from build123d import *

# Parameters (mm, degrees)
BOSS_EXTRUDE1_DEPTH = 30
SKETCH2_R           = 1.75
CUT_EXTRUDE2_DEPTH  = 42.231056256
CUT_EXTRUDE3_DEPTH  = 40.862263024
SKETCH5_W           = 33.611871568
SKETCH5_H           = 10
CUT_EXTRUDE4_DEPTH  = 42.231056256


with BuildPart() as part:
    # Sketch1 → Boss-Extrude1 (new body)
    with BuildSketch(Plane.XY):
        with BuildLine():
            Line((-20, 0), (-12.5, 0))
            ThreePointArc((-12.5, 0), (-10.752906584, 6.373774392), (-6, 10.9658561))
            Line((-6, 10.9658561), (6, 10.9658561))
            ThreePointArc((6, 10.9658561), (10.752906584, 6.373774392), (12.5, 0))
            Line((12.5, 0), (20, 0))
            ThreePointArc((20, 0), (0, 20), (-20, 0))
        make_face()
    extrude(amount=BOSS_EXTRUDE1_DEPTH)

    # Sketch2 → Cut-Extrude2 (cut, through all)
    with BuildSketch(Plane(origin=(0, 0, 0), x_dir=(1, 0, 0), z_dir=(0, 1, 0))):
        with Locations(Location((-17, -10, 0), (0, 0, 90))):
            Circle(SKETCH2_R)
        with Locations(Location((17, -10, 0), (0, 0, 90))):
            Circle(SKETCH2_R)
        with Locations(Location((17, -25, 0), (0, 0, 90))):
            Circle(SKETCH2_R)
        with Locations(Location((-17, -25, 0), (0, 0, 90))):
            Circle(SKETCH2_R)
    extrude(amount=CUT_EXTRUDE2_DEPTH, mode=Mode.SUBTRACT)

    # Sketch4 → Cut-Extrude3 (cut, through all)
    with BuildSketch(Plane(origin=(0, 3, 0), x_dir=(1, 0, 0), z_dir=(0, 1, 0))):
        Polygon((-17, -6.535898385), (-20, -8.267949192), (-20, -11.732050808), (-17, -13.464101615), (-14, -11.732050808), (-14, -8.267949192), align=None)
        Polygon((-17, -21.535898385), (-20, -23.267949192), (-20, -26.732050808), (-17, -28.464101615), (-14, -26.732050808), (-14, -23.267949192), align=None)
        Polygon((17, -21.535898385), (14, -23.267949192), (14, -26.732050808), (17, -28.464101615), (20, -26.732050808), (20, -23.267949192), align=None)
        Polygon((14, -8.267949192), (14, -11.732050808), (17, -13.464101615), (20, -11.732050808), (20, -8.267949192), (17, -6.535898385), align=None)
    extrude(amount=CUT_EXTRUDE3_DEPTH, mode=Mode.SUBTRACT)

    # Sketch5 → Cut-Extrude4 (cut, through all)
    with BuildSketch(Plane.XY.offset(30)):
        with Locations((0, 20)):
            Rectangle(SKETCH5_W, SKETCH5_H)
    extrude(amount=-CUT_EXTRUDE4_DEPTH, mode=Mode.SUBTRACT)


solid = part.part
Design review of the part built by this model. Coordinates are the model's own, in mm. A direction names the side the tool comes from. Coordinates: 2 decimals unless noted, no trailing zeros. Write each loop counter-clockwise with the first axis right and the second up, starting at its lowest first coordinate (ties: lowest second). Pieces come first, ordered by that corner, then holes. Notation, with made-up numbers: (64, 13) - (96, 13) arc R17 cw to (96, 43) - close; hole circle Ø6 at (-13, 0). An arc over 180 degrees is marked (long way). One line per item, written item: value.
1) Mouldability with a two-part tool opening along Z and no side actions: class faces 1 (the face through (18.1, 5.88, 7.17)), 2 (the face through (10.705, 6.454, 14.79)) as +Z half, -Z half, draft (parallel to the pull), parting line (faces both ways), or undercut.
Answer sheet:
face 1: undercut
face 2: draft
2) Add section D-D (x = 17.5). State the section outline as (y, z) points, plus the area to 3 significant figures.
Answer sheet:
outline: (0, 0) - (9.68, 0) - (9.68, 6.82) - (3, 6.82) - (3, 8.32) - (0, 8.32) - close; (0, 11.68) - (3, 11.68) - (3, 13.18) - (9.68, 13.18) - (9.68, 21.82) - (3, 21.82) - (3, 23.32) - (0, 23.32) - close; (0, 26.68) - (3, 26.68) - (3, 28.18) - (9.68, 28.18) - (9.68, 30) - (0, 30) - close
area: 185 mm2
3) Insertion check: pin 1 (4 mm diameter, centred on y = 11, z = 25, fed in from -X); pin 2 (4.5 mm diameter, centred on x = 16, z = 9.5, fed in from +Y); pin 3 (3 mm diameter, centred on x = -17, z = 25, fed in from -Y); pin 4 (3 mm diameter, centred on x = 17, z = 23.5, fed in from +Y). Each pin has a flat end and moves straight along its axis. Give the tip position at first contact, or say it passes through.
Answer sheet:
pin 1: stops at x = -14.46
pin 2: stops at y = 14.52
pin 3: passes through
pin 4: stops at y = 3
4) To check wall thickness, follow probe 1 along Z at (x, y) = (17, 1.6); probe 2 along X at (y, z) = (1.75, 25); probe 3 along X at (y, z) = (1.05, 10). State the ranges of each line that lie inside material, in increasing order.
Answer sheet:
probe 1: z = 0 to 8.25, 11.75 to 23.25, 26.75 to 30
probe 2: x = -19.92 to -18.75, -15.25 to -12.38, 12.38 to 15.25, 18.75 to 19.92
probe 3: x = -19.97 to -18.75, -15.25 to -12.46, 12.46 to 15.25, 18.75 to 19.97
5) Add section A-A (z = 10). State the section outline as (x, y) points.
Answer sheet:
outline: (-20, 0) - (-18.75, 0) - (-18.75, 3) - (-19.77, 3) arc R20 ccw to start; (-15.25, 0) - (-12.5, 0) arc R12.5 cw to (-6, 10.97) - (6, 10.97) arc R12.5 cw to (12.5, 0) - (15.25, 0) - (15.25, 3) - (14, 3) - (14, 14.28) arc R20 ccw to (13.23, 15) - (-13.23, 15) arc R20 ccw to (-14, 14.28) - (-14, 3) - (-15.25, 3) - close; (18.75, 0) - (20, 0) arc R20 ccw to (19.77, 3) - (18.75, 3) - close
6) Add section C-C (z = 15.5). State the section outline as (x, y) points.
Answer sheet:
outline: (-20, 0) - (-12.5, 0) arc R12.5 cw to (-6, 10.97) - (6, 10.97) arc R12.5 cw to (12.5, 0) - (20, 0) arc R20 ccw to (13.23, 15) - (-13.23, 15) arc R20 ccw to start
7) For faces 3 (the face through (14, 9, 25)), 4 (the face through (18.06, 5.88, 12.85)), 5 (the face through (-14, 9, 25)), list the 3-axis set-ups (+Z, -Z, +X, -X, +Y, -Y) from which the entire face can be reached by the end or side of a thin tool; tool diameter is ignored.
Answer sheet:
face 3: +X, +Y
face 4: +Y
face 5: -X, +Y
